The listing builds one solid part. Answer for the finished solid, in the listing's coordinates (mm). Face numbers are marked on the shaded views. A direction names the side the tool comes from. Coordinates: 2 decimals unless noted, no trailing zeros. Write each loop counter-clockwise with the first axis right and the second up, starting at its lowest first coordinate (ties: lowest second). Pieces come first, ordered by that corner, then holes. Notation, with made-up numbers: M 36,-36 L 62,-36 A11 ccw 62,-25 Z; hole C 31.5,62.5 d2. An arc over 180 degrees is marked long. Write item = value, one per line. Start each with the question number.
Autodesk Inventor part; units mm, degrees
ref_plane "YZ Plane" through (0, 0, 0) normal (1, 0, 0) x (0, 1, 0)
ref_plane "XZ Plane" through (0, 0, 0) normal (0, 1, 0) x (-1, 0, 0)
ref_plane "XY Plane" through (0, 0, 0) normal (0, 0, 1) x (1, 0, 0)
sketch "Sketch1" plane through (0, 0, 0) normal (0, 1, 0) x (-1, 0, 0)
  circle A0 centre (-218.3045, -174.8397) radius 152.4
  circle A1 centre (-218.3045, -174.8397) radius 114.3
  circle A2 centre (-218.3045, -174.8397) radius 57.15
  point P0 (0, 0)
  dimension "d0" = 304.8
  dimension "d1" = 228.6
  dimension "d6" = 114.3
extrude "Extrusion1" add sketch "Sketch1" along normal blind 63.5 contours A0
extrude "Extrusion2" add sketch "Sketch1" along normal blind 152.4 contours A1 | A2
sketch "Sketch2" plane through (218.3045, 152.4, -174.8397) normal (0, 1, 0) x (1, 0, 0)
  circle A0 centre (0, 0) radius 57.15
  point P0 (-218.3045, -174.8397)
  dimension "d7" = 114.3
extrude "Extrusion3" cut sketch "Sketch2" against normal through all
sketch "Sketch3" plane through (218.3045, 63.5, -174.8397) normal (0, 1, 0) x (1, 0, 0)
  circle A0 centre (133.5524, 0) radius 10.16
  circle A1 centre (0, 135.3792) radius 10.16
  circle A2 centre (-132.8036, 0) radius 10.16
  circle A3 centre (0, -134.7909) radius 11.3617
  point P0 (-218.3045, -174.8397)
  dimension "d10" = 20.32
  dimension "d11" = 20.32
  dimension "d12" = 20.32
properties part number "7.2 Part #"
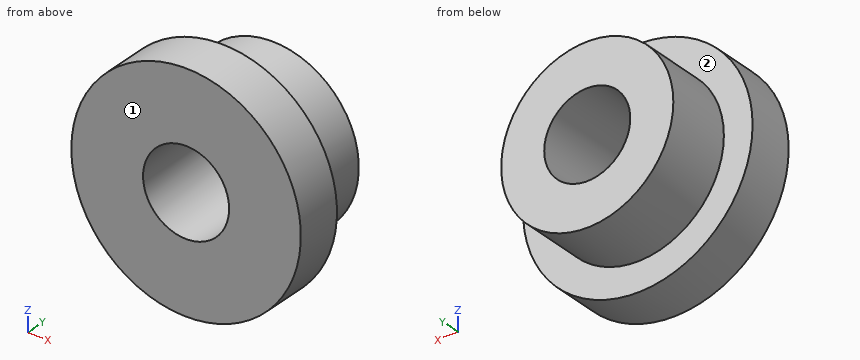
1. Straight lines are drawn through the part: L1, parallel to X at y = 49.5, z = -217; L2, parallel to Y at x = 277, z = -301.5; L3, parallel to Z at x = 189, y = 90. For each, find the intervals that lie inside material, in ascending order. Write a range as [from, to].
2. The part is cut by section A-A, the plane x = 244.5. Write down the section's boundary in (y, z).
3. For the marked faces 1 and 2, determine the directions among +Z, -Z, +X, -X, +Y, -Y from which every point of the face is accessible in a straight line to the end or side of a thin tool.
4. The part is cut by section C-C, the plane x = 121.5. Write down the section's boundary in (y, z).
5. The part is cut by section B-B, the plane z = -224. Write down the section's boundary in (x, y).
6. The part is cut by section D-D, the plane y = 31.5. Write down the section's boundary in (x, z).
7. Each of these flat-tipped pins is pushed along its axis until it touches: pin 1 (4 mm diameter, centred on x = 165.5, y = 78.5, fed in from +Z); pin 2 (1.5 mm diameter, centred on x = 323, y = 33.5, fed in from +Z); pin 3 (8 mm diameter, centred on y = 95.5, z = -121.5, fed in from -X). Where does it stop, or does it pass through?
Solution:
q1.L1 = [71.85, 179.72], [256.89, 364.76]
q1.L2 = [0, 63.5]
q1.L3 = [-285.32, -223.9], [-125.77, -64.36]
q2.outline = M 0,-324.97 L 63.5,-324.97 L 63.5,-286.1 L 152.4,-286.1 L 152.4,-225.63 L 0,-225.63 Z; M 0,-124.05 L 152.4,-124.05 L 152.4,-63.58 L 63.5,-63.58 L 63.5,-24.71 L 0,-24.71 Z
q3.face_1 = +Z, -Z, +X, -X, -Y
q3.face_2 = +Y
q4.outline = M 0,-292.55 L 63.5,-292.55 L 63.5,-235.61 L 152.4,-235.61 L 152.4,-114.07 L 63.5,-114.07 L 63.5,-57.13 L 0,-57.13 Z
q5.outline = M 74.05,0 L 189.16,0 L 189.16,152.4 L 115.12,152.4 L 115.12,63.5 L 74.05,63.5 Z; M 247.45,0 L 362.56,0 L 362.56,63.5 L 321.49,63.5 L 321.49,152.4 L 247.45,152.4 Z
q6.outline = C 218.3,-174.84 d304.8; hole C 218.3,-174.84 d114.3
q7.pin_1 = -72.45
q7.pin_2 = -63.39
q7.pin_3 = 115.2
